Build history of the part. All positions in model axes, mm. A direction names the side the tool comes from. Give positions to 0.01 mm unless a question says otherwise; leave off trailing zeros. Order: outer loops, then holes, each group sorted by start corner. A loop starts at its lowest first (then second) coordinate and runs counter-clockwise, first axis right, second up. Notation, with made-up numbers: (-29.75, 51.25) - (-7.75, 51.25) arc R12 ccw to (-7.75, 66.25) - close; hole circle Ø5 at (52, -16.75). An arc over 180 degrees is marked (long way). One line per item, written item: value.
Autodesk Inventor part; units mm, degrees
ref_plane "Work Plane1" through (64.5, 0, 0) normal (1, 0, 0) x (0, 0, -1)
ref_plane "Work Plane2" through (10.5, 0, 0) normal (-1, 0, 0) x (0, 0, 1)
ref_plane "YZ Plane" through (0, 0, 0) normal (1, 0, 0) x (0, 1, 0)
sketch "Sketch1" plane through (0, 0, 0) normal (0, 0, 1) x (1, 0, 0)
  line L0 (0, 0) -> (75, 0)
  line L1 (75, 0) -> (75, 30)
  line L2 (75, 30) -> (0, 30)
  line L3 (0, 30) -> (0, 0)
  point P0 (75, 15)
  point P1 (37.5, 30)
  dimension "d0" = 75
  dimension "d1" = 30
extrude "Extrusion1" add sketch "Sketch1" along normal blind 5
ref_plane "Work Plane1" through (64.5, 0, 0) normal (1, 0, 0) x (0, 0, -1)
sketch "Sketch2" plane through (64.5, 0, 0) normal (1, 0, 0) x (0, 0, -1)
  circle A0 centre (-10, 40) radius 4
  circle A1 centre (-10, 40) radius 7.5 construction
  arc A2 (-17.4763, 39.4047) -> (0, 0) centre (47.3186, 44.564) ccw
  arc A3 (-2.5195, 39.4597) -> (-17.4763, 39.4047) centre (-10, 40) ccw
  arc A4 (-2.5195, 39.4597) -> (0, 30) centre (12.4415, 38.379) ccw
  line L0 (0, 30) -> (-5, 30)
  line L1 (0, 0) -> (0, 30) construction
  line L2 (0, 30) -> (0, 0)
  dimension "d8" = 8
  dimension "d9" = 15
  dimension "d13" = 65
  dimension "d26" = 15
  dimension "d27" = 10
  dimension "d28" = 10
extrude "Extrusion2" add sketch "Sketch2" against normal blind 16.5
ref_plane "Work Plane2" through (10.5, 0, 0) normal (-1, 0, 0) x (0, 0, 1)
sketch "Sketch3" plane through (10.5, 0, 0) normal (-1, 0, 0) x (0, 0, 1)
  circle A0 centre (10, 40) radius 4
  line L0 (5, 5.9924) -> (5, 30)
  arc A1 (5, 5.9924) -> (17.4763, 39.4047) centre (-47.3186, 44.564) ccw
  arc A2 (17.4763, 39.4047) -> (2.5195, 39.4597) centre (10, 40) ccw
  line L1 (5, 30) -> (0, 30)
  arc A3 (0, 30) -> (2.5195, 39.4597) centre (-12.4415, 38.379) ccw
  point P0 (0, 0)
extrude "Extrusion3" add sketch "Sketch3" against normal blind 16.5
sketch "Sketch7" plane through (0, 0, 5) normal (0, 0, 1) x (1, 0, 0)
  line L0 (5, 15) -> (70, 15) construction
  line L1 (0, 0) -> (75, 0)
  circle A0 centre (5, 15) radius 2.5
  circle A1 centre (37.5, 15) radius 2.5
  circle A2 centre (70, 15) radius 2.5
  line L2 (0, 30) -> (0, 0)
  point P0 (37.5, 0)
  point P1 (0, 15)
  dimension "d29" = 65
  dimension "d30" = 5
  dimension "d31" = 5
  dimension "d32" = 5
extrude "Extrusion6" cut sketch "Sketch7" against normal through all
sketch "Sketch9" plane through (0, 0, 5) normal (0, 0, 1) x (1, 0, 0)
  line L0 (10.5, 30) -> (0, 30)
  line L1 (0, 30) -> (-5, 30)
  line L2 (-5, 30) -> (-5, 0)
  line L3 (-5, 0) -> (0, 0)
  line L4 (0, 0) -> (0, 30)
  line L5 (0, 0) -> (75, 0)
  line L6 (75, 0) -> (80, 0)
  line L7 (80, 0) -> (80, 30)
  line L8 (80, 30) -> (75, 30)
  line L9 (75, 30) -> (75, 0)
  point P0 (-2.5, 0)
  dimension "d37" = 5
  dimension "d38" = 5
extrude "Extrusion8" add sketch "Sketch9" against normal blind 5
sketch "Sketch8" plane through (10.5, 0, 0) normal (-1, 0, 0) x (0, 0, 1)
  arc A0 (5, 5.9924) -> (17.4763, 39.4047) centre (-47.3186, 44.564) ccw construction
  arc A1 (0, 0) -> (17.4763, 39.4047) centre (-47.3186, 44.564) ccw construction
  line L0 (5, 0) -> (5, 30)
  line L1 (5, 5.9924) -> (5, 0)
  line L2 (5, 0) -> (0, 0)
  arc A2 (0, 0) -> (5, 5.9924) centre (-47.3186, 44.564) ccw
extrude "Extrusion7" cut sketch "Sketch8" along normal through all both and the other way through all
properties part number "TC007b" material "ABS Plastic"
(1) Slice it at C-C, the plane z = 10. Give the cut face in (x, y), and give its area (3 significant figures).
Completed:
outline: (10.5, 13.91) - (27, 13.91) - (27, 36) - (10.5, 36) - close; (10.5, 44) - (27, 44) - (27, 47.5) - (10.5, 47.5) - close; (48, 13.91) - (64.5, 13.91) - (64.5, 36) - (48, 36) - close; (48, 44) - (64.5, 44) - (64.5, 47.5) - (48, 47.5) - close
area: 844 mm²
(2) Slice it at D-D, the plane y = 21. Give the cut face in (x, z), and give its area (3 significant figures).
Completed:
outline: (-5, 0) - (80, 0) - (80, 5) - (64.5, 5) - (64.5, 13.26) - (48, 13.26) - (48, 5) - (27, 5) - (27, 13.26) - (10.5, 13.26) - (10.5, 5) - (-5, 5) - close
area: 698 mm²
(3) Drill centre lines: line 1 (X direction, y = 26, z = 14.25); line 2 (Z direction, x = 44.5, y = 18); line 3 (Y direction, x = 18.5, z = 7.75). Where is each one in solid material? Low to high.
Completed:
line 1: 10.5 to 27, 48 to 64.5
line 2: 0 to 5
line 3: 10.03 to 36.69, 43.31 to 47.15
(4) Pull direction Y, two halves, no side cores. Call faces 5 (the face through (72, 30, 2)), 6 (the face through (64.5, 32, 9)), 7 (the face through (38.095, 2.963, 2.625)), 8 (the face through (7.31, 14.04, 2.54)): +Y half, -Y half, draft (parallel to the pull), parting line (faces both ways), or undercut.
Completed:
face 5: +Y half
face 6: draft
face 7: -Y half
face 8: undercut
(5) Pin check, flat tips, straight feed: P1, Ø5.5, axis at x = 2.5, z = 1.5, coming from the +Y side; P2, Ø3, axis at x = 5, y = 15, coming from the -Z side; P3, Ø5, axis at x = 64.5, z = 11.5, coming from the -Y side; P4, Ø8.5, axis at y = 34, z = 7, coming from the -X side. Stop position of each tip, or through.
Completed:
P1: y = 30
P2: through
P3: y = 12.11
P4: x = 10.5
(6) Slice it at B-B, the plane y = 15. Give the cut face in (x, z).
Completed:
outline: (-5, 0) - (2.5, 0) - (2.5, 5) - (-5, 5) - close; (7.5, 0) - (35, 0) - (35, 5) - (27, 5) - (27, 10.57) - (10.5, 10.57) - (10.5, 5) - (7.5, 5) - close; (40, 0) - (67.5, 0) - (67.5, 5) - (64.5, 5) - (64.5, 10.57) - (48, 10.57) - (48, 5) - (40, 5) - close; (72.5, 0) - (80, 0) - (80, 5) - (72.5, 5) - close
(7) 3-axis set-ups, long thin cutter, end or side, ignore diameter. For faces 1 (the face through (18.634, 21.589, 13.486)), 2 (the face through (48, 32, 9)), 3 (the face through (3, 18, 5)), 4 (the face through (47, 18, 5)): which of +Z, -Z, +X, -X, +Y, -Y reach the whole face in a straight line?
Completed:
face 1: +Z, +X, -X, -Y
face 2: +Z, +Y
face 3: +Z, -X, +Y, -Y
face 4: +Z, +Y, -Y
(8) Slice it at A-A, the plane x = 70. Give the cut face in (y, z), and give its area (3 significant figures).
Completed:
outline: (0, 0) - (12.5, 0) - (12.5, 5) - (5.99, 5) arc R65.01 ccw to start; (17.5, 0) - (30, 0) - (30, 5) - (17.5, 5) - close
area: 111 mm²
